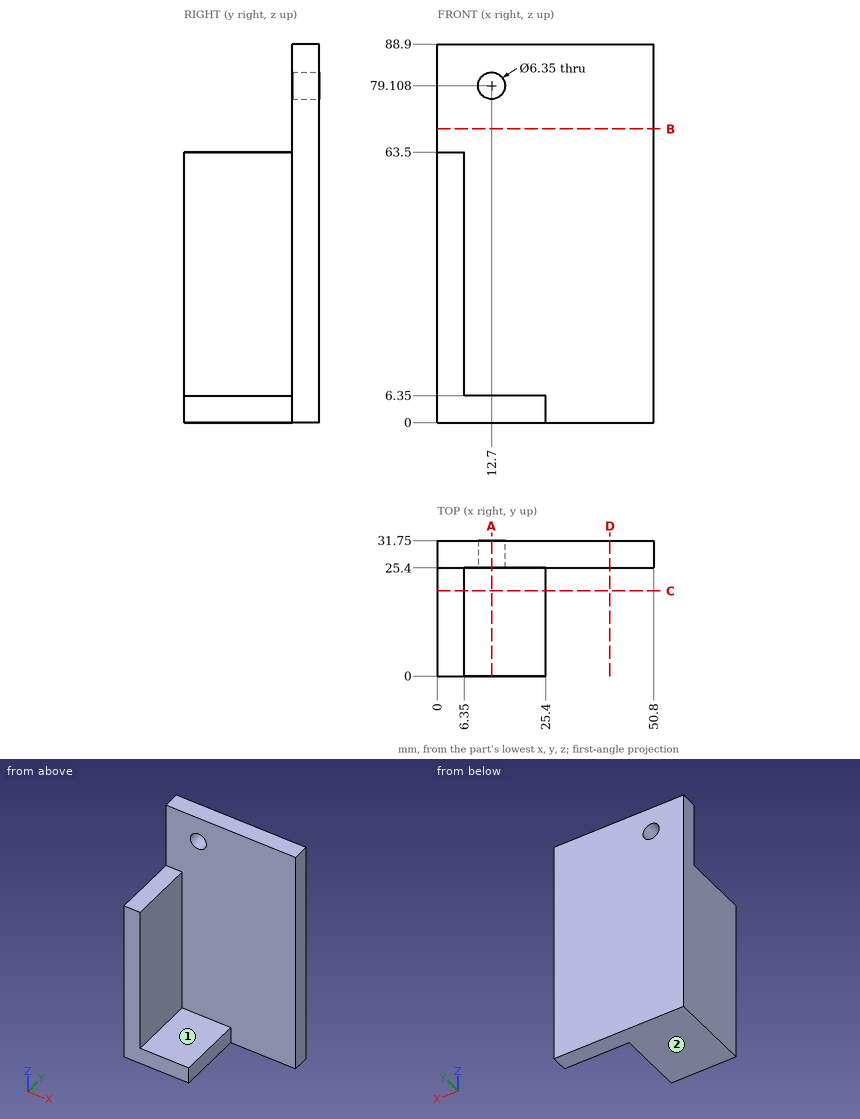
Geometry check sheet. Reference: drawing and pictorial views, mm from the part's lowest x, y, z. A direction names the side the tool comes from. Round coordinates to 2 decimals unless told otherwise and drop trailing zeros. Write each loop counter-clockwise with the first axis right and the second up, starting at its lowest first coordinate (ties: lowest second). Pieces come first, ordered by that corner, then holes.
Item 1: Section check C-C (y = 20). Record the boundary of the cut face in (x, z).
Determined:
outline: (0, 0) - (25.4, 0) - (25.4, 6.35) - (6.35, 6.35) - (6.35, 63.5) - (0, 63.5) - close
Item 2: Access from +Z, -Z, +X, -X, +Y, -Y to the whole of each face (thin tool, end or side, straight path). Record for the marked faces 1 and 2.
Determined:
face 1: +Z, +X, -Y
face 2: -Z, +X, -X, +Y, -Y
Item 3: Section check A-A (x = 12.7). Record the boundary of the cut face in (y, z).
Determined:
outline: (0, 0) - (31.75, 0) - (31.75, 75.93) - (25.4, 75.93) - (25.4, 6.35) - (0, 6.35) - close; (25.4, 82.28) - (31.75, 82.28) - (31.75, 88.9) - (25.4, 88.9) - close
Item 4: Material ranges on line 1 along Z through (x, y) = (12.7, 30); line 2 along Y through (x, z) = (37, 62); line 3 along X through (y, z) = (23, 59.5), recorded low to high.
Determined:
line 1: z = 0 to 75.93, 82.28 to 88.9
line 2: y = 25.4 to 31.75
line 3: x = 0 to 6.35
Item 5: Section check B-B (z = 69). Record the boundary of the cut face in (x, y).
Determined:
outline: (0, 25.4) - (50.8, 25.4) - (50.8, 31.75) - (0, 31.75) - close
Item 6: Section check D-D (x = 40.5). Record the boundary of the cut face in (y, z).
Determined:
outline: (25.4, 0) - (31.75, 0) - (31.75, 88.9) - (25.4, 88.9) - close
Item 7: Go/stop test with flat-tipped pins: pin 1 Ø5 at (x, y) = (13, 13) entering from +Z; pin 2 Ø8 at (y, z) = (13, 23.5) entering from +X; pin 3 Ø10 at (x, z) = (12.7, 79.11) entering from -Y. Record where each tip stops, or that it passes through.
Determined:
pin 1: stops at z = 6.35
pin 2: stops at x = 6.35
pin 3: stops at y = 25.4
